```python
from build123d import *

# Parameters (mm, degrees)
F0_W     = 76.2
F0_H     = 50.8
F1_DEPTH = 25.4
F3_DEPTH = 76.2
F4_R     = 5.08


with BuildPart() as f1:
    # F0 (on Front) → F1 (new body)
    with BuildSketch(Plane.XZ):
        with Locations((38.1, 25.4)):
            Rectangle(F0_W, F0_H)
    extrude(amount=F1_DEPTH)

    # F2 (on face) → F3 (join)
    with BuildSketch(Plane(origin=(0, 0, 0), x_dir=(-1, 0, 0), z_dir=(0, 1, 0))):
        Polygon((-43.975126, 9.23935), (-17.735837, 16.768539), (-24.533954, 35.03225), (-48.317943, 42.131286), (-66.098824, 27.070532), align=None)
    extrude(amount=F3_DEPTH)

    # F4
    f4_edges = [f1.edges().sort_by_distance(p)[0] for p in [
        (55.036975, 76.2, 18.154941),
        (30.855482, 76.2, 13.003944),
        (21.134895, 76.2, 25.900395),
        (36.425948, 76.2, 38.581768),
        (57.208383, 76.2, 34.600909),
    ]]
    fillet(f4_edges, radius=F4_R)


solid = f1.part
```
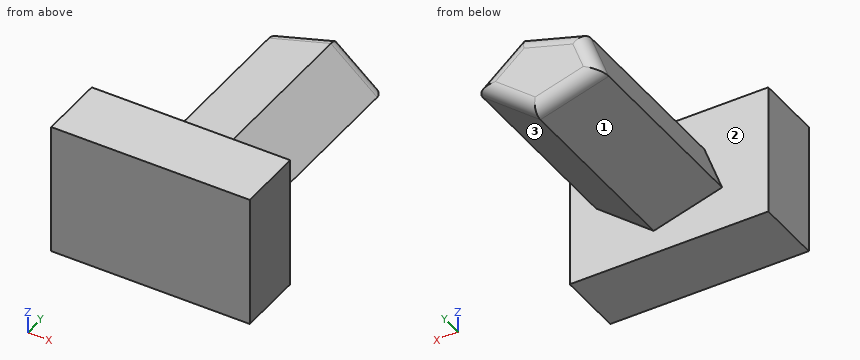
Geometry: final body of the model. Coordinates: model frame, mm. Face numbers are marked on the shaded views. A direction names the side the tool comes from. Coordinates: 2 decimals unless noted, no trailing zeros. Order: outer loops, then holes, each group sorted by start corner. A loop starts at its lowest first (then second) coordinate and runs counter-clockwise, first axis right, second up. Notation, with made-up numbers: M 39.5,64 L 43.5,64 A30 ccw 43.5,100 Z; hole C 50,78.5 d5. An arc over 180 degrees is marked long. Answer in a Markdown table with one row per item. Add a question column.
Q1. Section query A-A on y = 21. Return the cut outline in (x, z).
Q2. Reachability of the marked faces 1, 2 and 3 from +Z, -Z, +X, -X, +Y, -Y: full face, straight path, thin tool, end or side. Return the list, or none.
Q3. Line query: L1, parallel to Y at x = 56, z = 4; L2, parallel to Z at x = 48.5, y = 42; L3, parallel to Z at x = 40.5, y = 41. Output: solid intervals per line, ascending.
Q4. Section query C-C on z = 4. Return the cut outline in (x, y).
Q5. Contact query for flat-ended pins moving along their axis: P1, Ø4, axis at y = 38, z = 19, coming from the +X side; P2, Ø1.5, axis at x = 46, y = 45, coming from the -Z side; P3, Ø4, axis at x = 41.5, y = 63.5, coming from the +Z side. Output: stop coordinate, or through.
Q6. Section query B-B on x = 69.5. Return the cut outline in (y, z), and give its area (3 significant figures).
Completed:
| question | item | result |
|---|---|---|
| 1 | outline | M 17.74,16.77 L 43.98,9.24 L 66.1,27.07 L 48.32,42.13 L 24.53,35.03 Z |
| 2 | face 1 | -Z, -X, +Y |
| 2 | face 2 | +Y |
| 2 | face 3 | -Z, +X, +Y |
| 3 | L1 | y = -25.4 to 0 |
| 3 | L2 | z = 12.89 to 41.98 |
| 3 | L3 | z = 10.24 to 39.8 |
| 4 | outline | M 0,-25.4 L 76.2,-25.4 L 76.2,0 L 0,0 Z |
| 5 | P1 | stops at x = 58.57 |
| 5 | P2 | stops at z = 10.27 |
| 5 | P3 | stops at z = 40.69 |
| 6 | outline | M -25.4,0 L 0,0 L 0,50.8 L -25.4,50.8 Z |
| 6 | area | 1,290 mm2 |
